from build123d import *

# Parameters (mm, degrees)
EXTRUDE_THIN1_DEPTH = 182.7
SKETCH2_R           = 2.5
CUT_EXTRUDE1_DEPTH  = 120.738328299


with BuildPart() as part:
    # Sketch1 → Extrude-Thin1 (new body)
    with BuildSketch(Plane(origin=(0, 0, 0), x_dir=(0, 0, -1), z_dir=(1, 0, 0))):
        with BuildLine():
            Line((0.1, -47.818646587), (54.36916415, -47.818646587))
            ThreePointArc((54.36916415, -47.818646587), (57.904698056, -46.354180493), (59.36916415, -42.818646587))
            Line((59.36916415, -42.818646587), (59.36916415, 42.818646587))
            ThreePointArc((59.36916415, 42.818646587), (57.904698056, 46.354180493), (54.36916415, 47.818646587))
            Line((54.36916415, 47.818646587), (-54.36916415, 47.818646587))
            ThreePointArc((-54.36916415, 47.818646587), (-57.904698056, 46.354180493), (-59.36916415, 42.818646587))
            Line((-59.36916415, 42.818646587), (-59.36916415, -42.818646587))
            ThreePointArc((-59.36916415, -42.818646587), (-57.904698056, -46.354180493), (-54.36916415, -47.818646587))
            Line((-54.36916415, -47.818646587), (-0.1, -47.818646587))
            Line((-0.1, -47.818646587), (-0.1, -48.318646587))
            Line((-0.1, -48.318646587), (-54.36916415, -48.318646587))
            ThreePointArc((-54.36916415, -48.318646587), (-58.258251446, -46.707733884), (-59.86916415, -42.818646587))
            Line((-59.86916415, -42.818646587), (-59.86916415, 42.818646587))
            ThreePointArc((-59.86916415, 42.818646587), (-58.258251446, 46.707733884), (-54.36916415, 48.318646587))
            Line((-54.36916415, 48.318646587), (54.36916415, 48.318646587))
            ThreePointArc((54.36916415, 48.318646587), (58.258251446, 46.707733884), (59.86916415, 42.818646587))
            Line((59.86916415, 42.818646587), (59.86916415, -42.818646587))
            ThreePointArc((59.86916415, -42.818646587), (58.258251446, -46.707733884), (54.36916415, -48.318646587))
            Line((54.36916415, -48.318646587), (0.1, -48.318646587))
            Line((0.1, -48.318646587), (0.1, -47.818646587))
        make_face()
    extrude(amount=-EXTRUDE_THIN1_DEPTH)

    # Sketch2 → Cut-Extrude1 (cut, through all)
    with BuildSketch(Plane.XY.offset(59.86916415)):
        with Locations((-93.006946801, -6.886778216)):
            Circle(SKETCH2_R)
    extrude(amount=-CUT_EXTRUDE1_DEPTH, mode=Mode.SUBTRACT)


solid = part.part
Design review of the part built by this model. Coordinates are the model's own, in mm. A direction names the side the tool comes from. Round coordinates to 2 decimals unless told otherwise and drop trailing zeros. Write each loop counter-clockwise with the first axis right and the second up, starting at its lowest first coordinate (ties: lowest second). Pieces come first, ordered by that corner, then holes. Notation, with made-up numbers: (66.5, 64) -> (91.5, 64) arc R24 ccw to (91.5, 90) -> close; hole circle Ø11 at (11, 53.25). An arc over 180 degrees is marked (long way). One line per question, with ' | ' between items.
(1) Take a section at B-B, the plane y = -34. State the section outline as (x, z) points, and give its area (3 significant figures).
Result sheet:
outline: (-182.7, -59.87) -> (0, -59.87) -> (0, -59.37) -> (-182.7, -59.37) -> close; (-182.7, 59.37) -> (0, 59.37) -> (0, 59.87) -> (-182.7, 59.87) -> close | area: 183 mm2
(2) Draft analysis for pull direction Z (two halves, no side actions). For faces 3 (the flat face through (-90, -1, -59.369)), 4 (the flat face through (-90, 1, 59.369)), 5 (the cylindrical face through (-90.071, -46.665, -58.301)), 6 (the flat face through (-90, -1, 59.869)), state which applies: released by +Z, released by -Z, zero draft, split by the parting line, or undercut.
Result sheet:
face 3: undercut | face 4: undercut | face 5: released by -Z | face 6: released by +Z
(3) Take a section at A-A, the plane z = 25. State the section outline as (x, y) points.
Result sheet:
outline: (-182.7, -48.32) -> (0, -48.32) -> (0, -47.82) -> (-182.7, -47.82) -> close; (-182.7, 47.82) -> (0, 47.82) -> (0, 48.32) -> (-182.7, 48.32) -> close
(4) Take a section at C-C, the plane x = -137. State the section outline as (y, z) points.
Result sheet:
outline: (-48.32, -54.37) arc R5.5 ccw to (-42.82, -59.87) -> (42.82, -59.87) arc R5.5 ccw to (48.32, -54.37) -> (48.32, 54.37) arc R5.5 ccw to (42.82, 59.87) -> (-42.82, 59.87) arc R5.5 ccw to (-48.32, 54.37) -> (-48.32, 0.1) -> (-47.82, 0.1) -> (-47.82, 54.37) arc R5 cw to (-42.82, 59.37) -> (42.82, 59.37) arc R5 cw to (47.82, 54.37) -> (47.82, -54.37) arc R5 cw to (42.82, -59.37) -> (-42.82, -59.37) arc R5 cw to (-47.82, -54.37) -> (-47.82, -0.1) -> (-48.32, -0.1) -> close
(5) Insertion check: P1, Ø0.6, axis at x = -136.5, y = -48, coming from the +Z side; P2, Ø3, axis at x = -93.01, y = -6.89, coming from the -Z side; P3, Ø0.6, axis at x = -70, y = -48, coming from the -Z side. Each pin has a flat end and moves straight along its axis. Give the tip position at first contact, or say it passes through.
Result sheet:
P1: z = 56.9 | P2: through | P3: z = -56.9
(6) Wall thickness on line 1 (Y direction, x = -45, z = -4); line 2 (Z direction, x = -151, y = 20): over which ranges is each line inside the solid? List them lowest first. Write a range as [from, to].
Result sheet:
line 1: [-48.32, -47.82], [47.82, 48.32] | line 2: [-59.87, -59.37], [59.37, 59.87]
(7) Machinability: for faces 1 (the flat face through (-90, 47.819, -1)), 2 (the cylindrical face through (-90.071, 46.665, 58.301)), which of the approach directions +Z, -Z, +X, -X, +Y, -Y give a long, thin tool a straight path to every point of the face, cutting with its end or side? Answer none if there is none.
Result sheet:
face 1: +X, -X | face 2: +Z, +X, -X, +Y
